Geometry: final body of the model. Coordinates: model frame, mm. A direction names the side the tool comes from. Give positions to 0.01 mm unless a question says otherwise; leave off trailing zeros. Loops run counter-clockwise (first coordinate to the right, second up) from the corner with the lowest first, then second, coordinate; pieces in that order, holes last. Notation, with made-up numbers: M 5,-10 L 39,-10 A33 ccw 39,28 Z; hole C 51,52 d8. An arc over 180 degrees is marked long. Put each result on its own line as item: value.
```python
from build123d import *

# Parameters (mm, degrees)
SKETCH_1_W          = 54.5
SKETCH_1_H          = 32.5
EXTRUDE_2_DEPTH     = 34
EXTRUDE_3_DEPTH     = 5
EXTRUDE_6_DEPTH     = 4
SKETCH_14_W         = 46.9
SKETCH_14_H         = 28.7
CUT_EXTRUDE_6_DEPTH = 35
SKETCH_15_R         = 1.1
CUT_EXTRUDE_7_DEPTH = 47
EXTRUDE_7_DEPTH     = 2
SKETCH_18_R         = 8
CUT_EXTRUDE_8_DEPTH = 10
SKETCH_19_R         = 1
CUT_EXTRUDE_9_DEPTH = 20


with BuildPart() as part:
    # 草图1 → 凸台-拉伸2 (new body)
    with BuildSketch(Plane(origin=(0, 0, 0), x_dir=(1, 0, 0), z_dir=(0, 1, 0))):
        with Locations((4.534184514, 3.63509061)):
            Rectangle(SKETCH_1_W, SKETCH_1_H)
    extrude(amount=EXTRUDE_2_DEPTH)

    # 草图3 → 凸台-拉伸3 (add)
    with BuildSketch(Plane(origin=(0, 34, 0), x_dir=(1, 0, 0), z_dir=(0, 1, 0))):
        with BuildLine():
            Line((1.284184514, 34.88509061), (1.284184514, 19.88509061))
            Line((1.284184514, 19.88509061), (31.784184514, 19.88509061))
            Line((31.784184514, 19.88509061), (31.784184514, 34.88509061))
            ThreePointArc((31.784184514, 34.88509061), (16.534184514, 50.13509061), (1.284184514, 34.88509061))
        make_face()
    extrude_3 = extrude(amount=-EXTRUDE_3_DEPTH)

    # 草图11 → 凸台-拉伸6 (add)
    with BuildSketch(Plane.ZY.offset(-1.284184514)):
        Polygon((-34.88509061, 29), (-19.88509061, 17), (-19.88509061, 29), align=None)
    extrude_6 = extrude(amount=-EXTRUDE_6_DEPTH)

    # 镜向1: 凸台-拉伸3, 凸台-拉伸6 across plane
    add(extrude_3.mirror(Plane.ZY.offset(-16.534184514)))
    add(extrude_6.mirror(Plane.ZY.offset(-16.534184514)))

    # 草图14 → 切除-拉伸6 (cut, through all)
    with BuildSketch(Plane(origin=(0, 34, 0), x_dir=(1, 0, 0), z_dir=(0, 1, 0))):
        with Locations((4.534184514, 1.73509061)):
            Rectangle(SKETCH_14_W, SKETCH_14_H)
    extrude(amount=-CUT_EXTRUDE_6_DEPTH, mode=Mode.SUBTRACT)

    # 草图15 → 切除-拉伸7 (cut, symmetric)
    with BuildSketch(Plane.ZY.offset(-16.534184514)):
        with Locations((-9.63509061, 25.5)):
            Circle(SKETCH_15_R)
        with Locations((6.36490939, 25.5)):
            Circle(SKETCH_15_R)
    extrude(amount=CUT_EXTRUDE_7_DEPTH, both=True, mode=Mode.SUBTRACT)

    # 草图17 → 凸台-拉伸7 (add)
    with BuildSketch(Plane(origin=(0, 0, 0), x_dir=(1, 0, 0), z_dir=(0, 1, 0))):
        Polygon((-22.715815486, -12.61490939), (-22.715815486, 19.88509061), (31.784184514, 19.88509061), (31.784184514, -12.61490939), (27.984184514, -12.61490939), (27.984184514, 16.08509061), (-18.915815486, 16.08509061), (-18.915815486, -12.61490939), align=None)
    extrude(amount=-EXTRUDE_7_DEPTH)

    # 草图18 → 切除-拉伸8 (cut)
    with BuildSketch(Plane(origin=(0, 34, 0), x_dir=(1, 0, 0), z_dir=(0, 1, 0))):
        with Locations((16.534184514, 34.88509061)):
            Circle(SKETCH_18_R)
    extrude(amount=-CUT_EXTRUDE_8_DEPTH, mode=Mode.SUBTRACT)

    # 草图19 → 切除-拉伸9 (cut)
    with BuildSketch(Plane.XZ.offset(2)):
        with Locations((29.784184514, -17.88509061)):
            Circle(SKETCH_19_R)
        with Locations((-20.715815486, -17.88509061)):
            Circle(SKETCH_19_R)
    extrude(amount=-CUT_EXTRUDE_9_DEPTH, mode=Mode.SUBTRACT)


solid = part.part
```
Item 1: Pin query (flat end, axial travel): pin 1 Ø7.5 at (y, z) = (27, -31) entering from -X; pin 2 Ø5 at (x, y) = (25.5, 11.5) entering from -Z; pin 3 Ø0.6 at (x, z) = (29.5, -17.5) entering from -Y. Return the tip coordinate at first contact, or that it passes through.
Output values:
pin 1: x = 1.28
pin 2: z = -19.89
pin 3: y = 18
Item 2: Set-up query: faces 1 (the flat face through (27.984, 16, -2)), 2 (the flat face through (23, 29, -28)), 3 (the cylindrical face through (30.738, 7.86, -17.585)). Return all of +Z, -Z, +X, -X, +Y, -Y with unobstructed straight access to the full face (end or side cutting, diameter ignored); none if empty.
Output values:
face 1: +Z, +Y, -Y
face 2: -Z, -Y
face 3: -Y
Item 3: Section A-A on z = -12. Output: boundary loops of the cut face in (x, y), then the cut area to 3 significant figures.
Output values:
outline: M -22.72,-2 L -18.92,-2 L -18.92,34 L -22.72,34 Z; M 27.98,-2 L 31.78,-2 L 31.78,34 L 27.98,34 Z
area: 274 mm²
Item 4: Section B-B on y = 32. Output: boundary loops of the cut face in (x, z), then the cut area to 3 significant figures.
Output values:
outline: M -22.72,-19.89 L 1.28,-19.89 L 1.28,-34.89 A15.25 ccw 31.78,-34.89 L 31.78,12.61 L 27.98,12.61 L 27.98,-16.09 L -18.92,-16.09 L -18.92,12.61 L -22.72,12.61 Z; hole C 16.53,-34.89 d16
area: 1,050 mm²
Item 5: Line query: probe 1 along X at (y, z) = (-1, -5); probe 2 along Z at (x, y) = (-21, 25); probe 3 along Z at (x, y) = (29, 25). Output: solid intervals per line, ascending. Write a range as [from, to].
Output values:
probe 1: [-22.72, -18.92], [27.98, 31.78]
probe 2: [-19.89, -10.61], [-8.66, 5.39], [7.34, 12.61]
probe 3: [-29.89, -10.61], [-8.66, 5.39], [7.34, 12.61]
Item 6: Section C-C on x = 20.5. Output: boundary loops of the cut face in (y, z), then the cut area to 3 significant figures.
Output values:
outline: M -2,-19.89 L 29,-19.89 L 29,-27.94 L 34,-27.94 L 34,-16.09 L -2,-16.09 Z; M 29,-49.61 L 34,-49.61 L 34,-41.83 L 29,-41.83 Z
area: 216 mm²
Item 7: Mould query, pull axis X, two halves, no side actions, for faces 4 (the flat face through (-21, 16, 12.615)), 5 (the flat face through (-22.716, 16, -3)), 6 (the cylindrical face through (15.493, 31.535, -42.817)), 7 (the flat face through (5, 16, -16.085)). Classes: pulls with the +X half, pulls with the -X half, needs draft (parallel to the pull), parting line crosses it, or undercut.
Output values:
face 4: needs draft
face 5: pulls with the -X half
face 6: undercut
face 7: undercut
Item 8: Section D-D on y = 25.5. Count the separate pieces of the cut face and the enclosed holes in it, then the cut area to 3 significant figures.
Output values:
separate pieces: 5
enclosed holes: 0
area: 477 mm²
